from build123d import *

# Parameters (mm, degrees)
ESBO_O1_W                = 71.15
ESBO_O1_H                = 72
RESSALTO_EXTRUS_O1_DEPTH = 1.5
ESBO_O2_W                = 66.75
ESBO_O2_H                = 67.6
ESBO_O2_W_2              = 62.15
ESBO_O2_H_2              = 63
RESSALTO_EXTRUS_O2_DEPTH = 8
FILETE1_R                = 2
ESBO_O3_W                = 9
ESBO_O3_H                = 8
CORTE_EXTRUS_O1_DEPTH    = 4.5
ESBO_O4_W                = 8.5
ESBO_O4_H                = 8
CORTE_EXTRUS_O2_DEPTH    = 4.5
ESBO_O5_W                = 15
ESBO_O5_H                = 8
CORTE_EXTRUS_O3_DEPTH    = 4.5


with BuildPart() as part:
    # Esboço1 → Ressalto-extrusão1 (new body, symmetric)
    with BuildSketch(Plane(origin=(0, 0, 0), x_dir=(1, 0, 0), z_dir=(0, 1, 0))):
        Rectangle(ESBO_O1_W, ESBO_O1_H)
    extrude(amount=RESSALTO_EXTRUS_O1_DEPTH, both=True)

    # Esboço2 → Ressalto-extrusão2 (add)
    with BuildSketch(Plane(origin=(0, 1.5, 0), x_dir=(1, 0, 0), z_dir=(0, 1, 0))):
        Rectangle(ESBO_O2_W, ESBO_O2_H)
        Rectangle(ESBO_O2_W_2, ESBO_O2_H_2, mode=Mode.SUBTRACT)
    extrude(amount=RESSALTO_EXTRUS_O2_DEPTH)

    # Filete1
    filete1_edges = [part.edges().sort_by_distance(p)[0] for p in [
        (-33.375, 5.5, 33.8),
        (33.375, 5.5, 33.8),
        (33.375, 5.5, -33.8),
        (-33.375, 5.5, -33.8),
        (35.575, 0, 36),
        (-35.575, 0, 36),
        (-35.575, 0, -36),
        (35.575, 0, -36),
    ]]
    fillet(filete1_edges, radius=FILETE1_R)

    # Esboço3 → Corte-extrusão1 (cut)
    with BuildSketch(Plane.ZY.offset(-31.075)):
        with Locations((-13, 5.5)):
            Rectangle(ESBO_O3_W, ESBO_O3_H)
    extrude(amount=-CORTE_EXTRUS_O1_DEPTH, mode=Mode.SUBTRACT)

    # Esboço4 → Corte-extrusão2 (cut)
    with BuildSketch(Plane.ZY.offset(-31.075)):
        with Locations((-2.25, 5.5)):
            Rectangle(ESBO_O4_W, ESBO_O4_H)
    extrude(amount=-CORTE_EXTRUS_O2_DEPTH, mode=Mode.SUBTRACT)

    # Esboço5 → Corte-extrusão3 (cut)
    with BuildSketch(Plane(origin=(0, 0, 31.5), x_dir=(-1, 0, 0), z_dir=(0, 0, -1))):
        with Locations((-9.225, 5.5)):
            Rectangle(ESBO_O5_W, ESBO_O5_H)
    extrude(amount=-CORTE_EXTRUS_O3_DEPTH, mode=Mode.SUBTRACT)


solid = part.part
Work out the finished part from the listing and answer in its coordinate system (mm). A direction names the side the tool comes from. Give positions to 0.01 mm unless a question says otherwise; leave off trailing zeros. Write each loop counter-clockwise with the first axis right and the second up, starting at its lowest first coordinate (ties: lowest second). Pieces come first, ordered by that corner, then holes. Notation, with made-up numbers: (-32, 85.25) - (20, 85.25) arc R23 cw to (20, 100.25) - close; hole circle Ø7 at (62.5, 33). An arc over 180 degrees is marked (long way). One line per item, written item: value. Start each with the question number.
1. For a pull along Z with two mould halves and no side action, classify faces 4 (the cylindrical face through (-35.005, 0.021, 35.399)), 5 (the flat face through (-31.075, 5, 0)), 6 (the flat face through (32, 9.5, 21)) as +Z half, -Z half, draft (parallel to the pull), parting line (faces both ways), or undercut.
2. Consider probe 1 along X at (y, z) = (2, 16.5) (3 decimals); probe 2 along Z at (x, y) = (-29, 3.5); probe 3 along Y at (x, z) = (19, -23.5). Determine where each line is inside the solid, lowest interval first.
3. Find section C-C (x = 13.5). Write down the section's boundary in (y, z).
4. Given pin 1 (6.5 mm diameter, centred on y = 6, z = -22.5, fed in from +X) (3 decimals); pin 2 (12 mm diameter, centred on x = 18.5, z = -3.5, fed in from +Y); pin 3 (2.5 mm diameter, centred on y = 3.5, z = 15, fed in from -X) (3 decimals), each flat-ended and moving along its own axis, determine where each tip first touches the part or whether it passes through.
5. For faces 1 (the flat face through (24, 5, 31.5)), 2 (the flat face through (32, 5, -17.5)), 3 (the cylindrical face through (32.774, 5.556, 33.23)), determine the directions among +Z, -Z, +X, -X, +Y, -Y from which every point of the face is accessible in a straight line to the end or side of a thin tool.
6. Find section D-D (z = -19). Write down the section's boundary in (x, y) (3 decimals).
7. Find section B-B (z = -2.5). Write down the section's boundary in (x, y) (3 decimals), then the cut area to 3 significant figures.
8. Find section A-A (y = 2.5). Write down the section's boundary in (x, z) (3 decimals), then the cut area to 3 significant figures.
Geometry results:
1. face 4: +Z half
1. face 5: undercut
1. face 6: draft
2. probe 1: -33.375 to -31.075, 31.075 to 33.375
2. probe 2: -33.8 to -31.5, 31.5 to 33.8
2. probe 3: -1.5 to 1.5
3. outline: (-1.5, -36) - (1.5, -36) - (1.5, -33.8) - (9.5, -33.8) - (9.5, -31.5) - (1.5, -31.5) - (1.5, 36) - (-1.5, 36) - close
4. pin 1: x = 33.375
4. pin 2: y = 1.5
4. pin 3: x = -33.375
5. face 1: +Y
5. face 2: +X, +Y
5. face 3: +Z, +X, +Y
6. outline: (-35.575, -1.5) - (35.575, -1.5) - (35.575, 1.5) - (33.375, 1.5) - (33.375, 9.5) - (31.075, 9.5) - (31.075, 1.5) - (-31.075, 1.5) - (-31.075, 9.5) - (-33.375, 9.5) - (-33.375, 1.5) - (-35.575, 1.5) - close
7. outline: (-35.575, -1.5) - (35.575, -1.5) - (35.575, 1.5) - (-31.075, 1.5) - (-31.075, 9.5) - (-33.375, 9.5) - (-33.375, 1.5) - (-35.575, 1.5) - close
7. area: 232 mm2
8. outline: (-33.375, -31.8) arc R2 ccw to (-31.375, -33.8) - (31.375, -33.8) arc R2 ccw to (33.375, -31.8) - (33.375, -17.5) - (31.075, -17.5) - (31.075, -31.5) - (-31.075, -31.5) - (-31.075, 31.5) - (1.725, 31.5) - (1.725, 33.8) - (-31.375, 33.8) arc R2 ccw to (-33.375, 31.8) - close; (16.725, 31.5) - (31.075, 31.5) - (31.075, 2) - (33.375, 2) - (33.375, 31.8) arc R2 ccw to (31.375, 33.8) - (16.725, 33.8) - close; (31.075, -8.5) - (33.375, -8.5) - (33.375, -6.5) - (31.075, -6.5) - close
8. area: 519 mm2
